Part print with two shaded views. Sizes in mm from the minimum x, y, z corner. A direction names the side the tool comes from. Round coordinates to 2 decimals unless told otherwise and drop trailing zeros. Write each loop counter-clockwise with the first axis right and the second up, starting at its lowest first coordinate (ties: lowest second). Pieces come first, ordered by that corner, then holes. Notation, with made-up numbers: (31.25, 5) -> (54.25, 5) arc R34 ccw to (54.25, 39) -> close; hole circle Ø5 at (53.25, 21.5). An arc over 180 degrees is marked (long way). Answer in a Markdown table with one row per item.
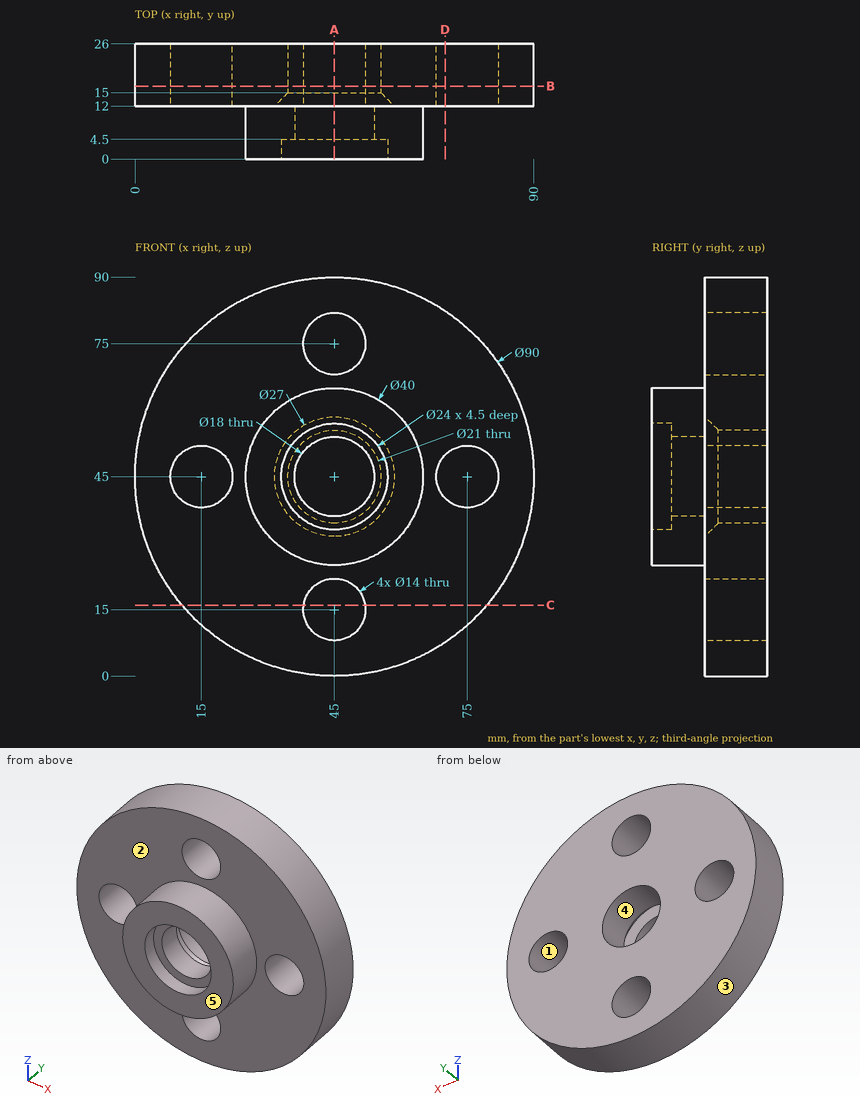
Q1. Wall check: line 1 (X direction, y = 23.25, z = 48); line 2 (X direction, y = 7, z = 45); line 3 (X direction, y = 13.25, z = 41). Give the ranges that are in metal, low to high. Write a range as [from, to].
A:
| item | result |
|---|---|
| line 1 | [0.1, 8.68], [21.32, 34.94], [55.06, 68.68], [81.32, 89.9] |
| line 2 | [25, 36], [54, 65] |
| line 3 | [0.18, 9.26], [20.74, 33.42], [56.58, 69.26], [80.74, 89.82] |
Q2. Saw through at C-C on z = 16. Write the cut outline in (x, y), plus the area to 3 significant figures.
A:
| item | result |
|---|---|
| outline | (10.59, 12) -> (38.07, 12) -> (38.07, 26) -> (10.59, 26) -> close; (51.93, 12) -> (79.41, 12) -> (79.41, 26) -> (51.93, 26) -> close |
| area | 769 mm² |
Q3. Drop flat-ended pins along their axis: P1, Ø10, axis at y = 13, z = 10.5, coming from the -X side; P2, Ø7, axis at x = 46.5, z = 41, coming from the -Y side; P3, Ø2, axis at x = 53, z = 46.5, coming from the -Y side; P4, Ø1, axis at x = 61.5, z = 23.5, coming from the -Y side. Give the stop position or say it passes through.
A:
| item | result |
|---|---|
| P1 | x = 11.02 |
| P2 | through |
| P3 | y = 4.5 |
| P4 | y = 12 |
Q4. Two-plate mould, pull along Z, no slides. Class the marked faces 3, 4 and 5: released by +Z, released by -Z, zero draft, split by the parting line, or undercut.
A:
| item | result |
|---|---|
| face 3 | split by the parting line |
| face 4 | undercut |
| face 5 | zero draft |
Q5. Saw through at A-A on x = 45. State how many separate pieces and enclosed holes the cut face has, plus the area to 3 significant figures.
A:
| item | result |
|---|---|
| separate pieces | 4 |
| enclosed holes | 0 |
| area | 802 mm² |
Q6. Saw through at D-D on x = 70. Write the cut outline in (y, z).
A:
| item | result |
|---|---|
| outline | (12, 7.58) -> (26, 7.58) -> (26, 40.1) -> (12, 40.1) -> close; (12, 49.9) -> (26, 49.9) -> (26, 82.42) -> (12, 82.42) -> close |
Q7. Which spindle directions (+Z, -Z, +X, -X, +Y, -Y) get a long thin tool onto all of the face, cutting with end or side? Do the marked faces 1 and 2. Say none if no direction does.
A:
| item | result |
|---|---|
| face 1 | +Y, -Y |
| face 2 | -Y |
Q8. Saw through at B-B on y = 16.5. Write the cut outline in (x, z).
A:
| item | result |
|---|---|
| outline | circle Ø90 at (45, 45); hole circle Ø14 at (15, 45); hole circle Ø21 at (45, 45); hole circle Ø14 at (45, 15); hole circle Ø14 at (45, 75); hole circle Ø14 at (75, 45) |
